Autodesk Inventor part; units mm, degrees
ref_plane "YZ Plane" through (0, 0, 0) normal (1, 0, 0) x (0, 1, 0)
ref_plane "XZ Plane" through (0, 0, 0) normal (0, 1, 0) x (-1, 0, 0)
ref_plane "XY Plane" through (0, 0, 0) normal (0, 0, 1) x (1, 0, 0)
sketch "Sketch1" plane through (0, 0, 0) normal (1, 0, 0) x (0, 1, 0)
  line L0 (0, 0) -> (3.175, 0)
  line L1 (3.175, 0) -> (3.175, -50.8)
  line L2 (3.175, -50.8) -> (0, -50.8)
  line L3 (0, -50.8) -> (0, 0)
  line L4 (0, 0) -> (50.8, 0)
  line L5 (50.8, 0) -> (50.8, -3.175)
  line L6 (50.8, -3.175) -> (0, -3.175)
  line L7 (0, -3.175) -> (0, 0)
  dimension "d0" = 3.175
  dimension "d1" = 50.8
  dimension "d2" = 50.8
  dimension "d3" = 3.175
extrude "Extrusion1" add sketch "Sketch1" along normal blind 469.9
sketch "Sketch2" plane through (0, 0, -50.8) normal (0, -1, 0) x (1, 0, 0)
  line L0 (469.9, 50.8) -> (469.9, 0)
  line L1 (0, 50.8) -> (469.9, 50.8)
  line L2 (0, 50.8) -> (0, 0)
  line L3 (0, 0) -> (469.9, 0)
  point P0 (12.7, 41.275)
  point P1 (12.7, 15.875)
  point P2 (457.2, 41.275)
  point P3 (457.2, 15.875)
  dimension "d6" = 12.7
  dimension "d7" = 9.525
  dimension "d8" = 15.875
  dimension "d9" = 12.7
  dimension "d10" = 12.7
  dimension "d11" = 9.525
  dimension "d12" = 12.7
  dimension "d13" = 15.875
hole "Hole1" at (12.7, 0, -9.525) at (12.7, 0, -34.925) at (457.2, 0, -9.525) at (457.2, 0, -34.925) direction (0, 1, 0) diameter 6.35 end through all
sketch "Sketch3" plane through (0, 0, 0) normal (-1, 0, 0) x (0, 0, 1)
  line L0 (0, 0) -> (-50.8, 0)
  line L1 (0, 50.8) -> (0, 0)
  line L2 (-3.175, 50.8) -> (0, 50.8)
  line L3 (-3.175, 3.175) -> (-3.175, 50.8)
  line L4 (-50.8, 3.175) -> (-3.175, 3.175)
  line L5 (-50.8, 0) -> (-50.8, 3.175)
  line L6 (0, 50.8) -> (-3.175, 50.8)
  line L7 (-3.175, 50.8) -> (-3.175, 25.4)
  line L8 (-3.175, 25.4) -> (0, 25.4)
  line L9 (0, 25.4) -> (0, 50.8)
  dimension "d21" = 3.175
  dimension "d22" = 25.4
extrude "Extrusion2" cut sketch "Sketch3" against normal blind 660.4 contours L8 L3 L2 L1
properties part number "2x2 angle horizontal"
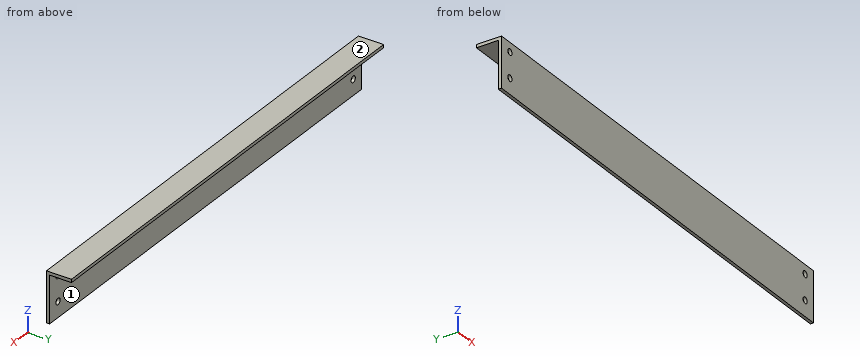
Can you work these out from the model? Positions are in its coordinate system, mm. Face numbers are marked on the shaded views. A direction names the side the tool comes from. Coordinates: 2 decimals unless noted, no trailing zeros. Loops run counter-clockwise (first coordinate to the right, second up) from the corner with the lowest first, then second, coordinate; pieces in that order, holes last. Notation, with made-up numbers: (70.5, 44) - (100.5, 44) arc R23 cw to (100.5, 76) - close; hole circle Ø7 at (50, 12). An arc over 180 degrees is marked (long way). Use a Markdown table: item, result.
Item 1: Will these pins go through, and if not, where does the flat tip stop? pin 1 (4 mm diameter, centred on x = 92, y = 15.5, fed in from +Z); pin 2 (4 mm diameter, centred on x = 325, z = -28, fed in from +Y) (3 decimals); pin 3 (6.5 mm diameter, centred on x = 290, y = 14.5, fed in from -Z) (3 decimals).
Numbers:
| item | result |
|---|---|
| pin 1 | stops at z = 0 |
| pin 2 | stops at y = 3.175 |
| pin 3 | stops at z = -3.175 |
Item 2: I want a section at C-C on z = -25. Please give me the cut outline in (x, y) (3 decimals), and give its area (3 significant figures).
Numbers:
| item | result |
|---|---|
| outline | (0, 0) - (469.9, 0) - (469.9, 3.175) - (0, 3.175) - close |
| area | 1,490 mm2 |
Item 3: I want a section at A-A on x = 197. Please give me the cut outline in (y, z) (3 decimals).
Numbers:
| item | result |
|---|---|
| outline | (0, -50.8) - (3.175, -50.8) - (3.175, -3.175) - (25.4, -3.175) - (25.4, 0) - (0, 0) - close |
Item 4: For the marked faces 1 and 2, which set-ups out of +Z, -Z, +X, -X, +Y, -Y let a thin tool reach every point of the face, with its end or its side?
Numbers:
| item | result |
|---|---|
| face 1 | -Z, +X, -X, +Y |
| face 2 | +Z, +X, -X, +Y, -Y |
Item 5: I want a section at B-B on y = 14. Please give me the cut outline in (x, z) (3 decimals), and give its area (3 significant figures).
Numbers:
| item | result |
|---|---|
| outline | (0, -3.175) - (469.9, -3.175) - (469.9, 0) - (0, 0) - close |
| area | 1,490 mm2 |
Item 6: If I drill on probe 1 along Z at (x, y) = (457.2, 0.7); probe 2 along X at (y, z) = (1.5, -32); probe 3 along Y at (x, z) = (423.5, -37.5) (3 decimals), over which ranges is the centre line in solid material (lowest first)? Write a range as from..to.
Numbers:
| item | result |
|---|---|
| probe 1 | z = -50.8..-38.1, -31.75..-12.7, -6.35..0 |
| probe 2 | x = 0..11.47, 13.93..455.97, 458.43..469.9 |
| probe 3 | y = 0..3.175 |
